Can you work these out from the drawing? Everything is in mm from the part's minimum corner. Give positions to 0.01 mm unless a question says otherwise; leave off trailing zeros. Loops run counter-clockwise (first coordinate to the right, second up) from the corner with the lowest first, then second, coordinate; pieces in that order, holes last. Notation, with made-up numbers: (-30.75, 66.5) - (23.25, 66.5) arc R20 ccw to (23.25, 80.5) - close; hole circle Ø1 at (-19, -18). An arc over 180 degrees is marked (long way). One line per item, written item: value. Start each with the question number.
Q1. I want a section at A-A (z = 1.4). Please give me the cut outline in (x, y).
Q2. If I drill on line 1 (Z direction, x = 2.35, y = 14) (1 decimal); line 2 (X direction, y = 3.25, z = 2.45) (1 decimal); line 3 (X direction, y = 10.75, z = 1.95) (1 decimal), over which ranges is the centre line in solid material (lowest first)? Write a range as from..to.
Q3. I want a section at C-C (x = 2.9). Please give me the cut outline in (y, z).
Q4. If we mould it in two halves opening along Z, with no side actions, what happens to the marked faces 1, 2, 3 and 4? For each: released by +Z, released by -Z, zero draft, split by the parting line, or undercut.
Q5. I'm going to push a flat-ended pin straight in: P1, Ø2, axis at y = 2, z = 3.5, coming from the +X side (1 decimal). Where does the tip first touch, or does it pass through?
Q6. I want a section at D-D (z = 0.3). Please give me the cut outline in (x, y) (1 decimal).
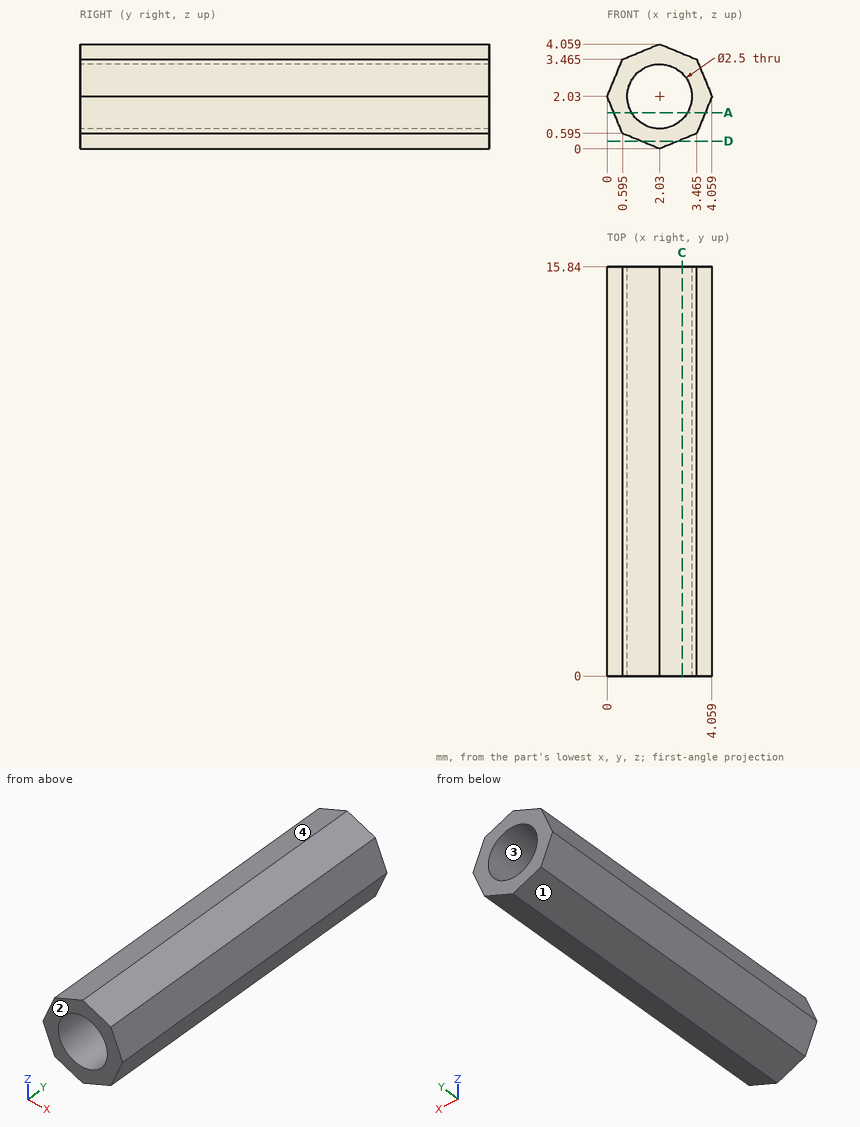
Worked answers:
1. outline: (0.26, 0) - (0.95, 0) - (0.95, 15.84) - (0.26, 15.84) - close; (3.11, 0) - (3.8, 0) - (3.8, 15.84) - (3.11, 15.84) - close
2. line 1: z = 0.1..0.8, 3.2..3.9
2. line 2: x = 0.2..0.9, 3.2..3.9
2. line 3: x = 0..0.8, 3.3..4
3. outline: (0, 0.36) - (15.84, 0.36) - (15.84, 1.13) - (0, 1.13) - close; (0, 2.93) - (15.84, 2.93) - (15.84, 3.7) - (0, 3.7) - close
4. face 1: released by -Z
4. face 2: zero draft
4. face 3: undercut
4. face 4: released by +Z
5. P1: stops at x = 3.9
6. outline: (1.3, 0) - (2.8, 0) - (2.8, 15.8) - (1.3, 15.8) - close
